from build123d import *

# Parameters (mm, degrees)
SKETCH1_W               = 19.05
SKETCH1_H               = 19.05
SKETCH1_W_2             = 15.875
SKETCH1_H_2             = 15.875
BOSS_EXTRUDE1_DEPTH     = 196.85
CUT_EXTRUDE1_DEPTH      = 198.310348816
CUT_EXTRUDE1_DEPTH_BACK = 198.310348816
SKETCH2_R               = 6.35


with BuildPart() as part:
    # Sketch1 → Boss-Extrude1 (new, symmetric)
    with BuildSketch(Plane.XY):
        Rectangle(SKETCH1_W, SKETCH1_H)
        Rectangle(SKETCH1_W_2, SKETCH1_H_2, mode=Mode.SUBTRACT)
    extrude(amount=BOSS_EXTRUDE1_DEPTH, both=True)

    # Sketch2 → Cut-Extrude1 (cut, two sides: drawn at the far end of the back side and taken through both)
    with BuildSketch(Plane(origin=(0, 0, 0), x_dir=(0, 0, -1), z_dir=(1, 0, 0)).offset(-CUT_EXTRUDE1_DEPTH_BACK)):
        Circle(SKETCH2_R)
    extrude(amount=CUT_EXTRUDE1_DEPTH + CUT_EXTRUDE1_DEPTH_BACK, mode=Mode.SUBTRACT)


solid = part.part
For this review, take the finished solid that the model builds, in its own axes (mm). A direction names the side the tool comes from. Round coordinates to 2 decimals unless told otherwise and drop trailing zeros. Order: outer loops, then holes, each group sorted by start corner. A loop starts at its lowest first (then second) coordinate and runs counter-clockwise, first axis right, second up. Notation, with made-up numbers: (40, 28) -> (85, 28) arc R31 ccw to (85, 54) -> close; hole circle Ø6 at (81, 83.5). An arc over 180 degrees is marked (long way). Put each result on its own line as item: value.
Q1. Machinability: for faces 1 (the flat face through (9.525, 6, 3)), 2 (the flat face through (7.938, 7, 3)), which of the approach directions +Z, -Z, +X, -X, +Y, -Y give a long, thin tool a straight path to every point of the face, cutting with its end or side? Answer none if there is none.
Check result:
face 1: +Z, -Z, +X, +Y, -Y
face 2: +Z, -Z
Q2. Add section A-A on y = 0. State how many separate pieces and enclosed holes the cut face has, plus the area to 3 significant figures.
Check result:
separate pieces: 4
enclosed holes: 0
area: 1,210 mm2
Q3. Add section D-D on z = -171. Write out the cut boundary in (x, y) (1 decimal).
Check result:
outline: (-9.5, -9.5) -> (9.5, -9.5) -> (9.5, 9.5) -> (-9.5, 9.5) -> close; hole (-7.9, -7.9) -> (7.9, -7.9) -> (7.9, 7.9) -> (-7.9, 7.9) -> close
Q4. Mouldability with a two-part tool opening along Z and no side actions: class faces 3 (the flat face through (-9, 0, 196.85)), 4 (the flat face through (0, 7.938, 3)), 5 (the cylindrical face through (8.72, -6.2, 1.38)), 6 (the cylindrical face through (-8.74, -6.2, 1.38)) as pulls with the +Z half, pulls with the -Z half, needs draft (parallel to the pull), parting line crosses it, or undercut.
Check result:
face 3: pulls with the +Z half
face 4: needs draft
face 5: undercut
face 6: undercut
Q5. For probe 1 along X at (y, z) = (4, 51) (1 decimal); probe 2 along Z at (x, y) = (-8.9, 0), list the stretches that pass through material, from the lowest coordinate up. Write a range as [from, to].
Check result:
probe 1: [-9.5, -7.9], [7.9, 9.5]
probe 2: [-196.85, -6.35], [6.35, 196.85]
